from build123d import *

# Parameters (mm, degrees)
F1_DEPTH = 3


with BuildPart() as f1:
    # F0 (on Top) → F1 (new body)
    with BuildSketch(Plane.XY):
        with BuildLine():
            Line((-21, 3.2), (-21, 0))
            ThreePointArc((-21, 0), (-20.124574, -6.000127), (-17.571283, -11.5))
            ThreePointArc((-17.571283, -11.5), (-13.499794, -16.085881), (-8.277077, -19.3))
            Line((-8.277077, -19.3), (8.277077, -19.3))
            ThreePointArc((8.277077, -19.3), (13.499794, -16.085881), (17.571283, -11.5))
            ThreePointArc((17.571283, -11.5), (20.124574, -6.000127), (21, 0))
            Line((21, 0), (19, 0))
            Line((19, 0), (19, 3.2))
            Line((19, 3.2), (11, 3.2))
            Line((11, 3.2), (11, 0))
            Line((11, 0), (3, 0))
            Line((3, 0), (3, 3.2))
            Line((3, 3.2), (-5, 3.2))
            Line((-5, 3.2), (-5, 0))
            Line((-5, 0), (-13, 0))
            Line((-13, 0), (-13, 3.2))
            Line((-13, 3.2), (-21, 3.2))
        make_face()
    extrude(amount=F1_DEPTH)


solid = f1.part
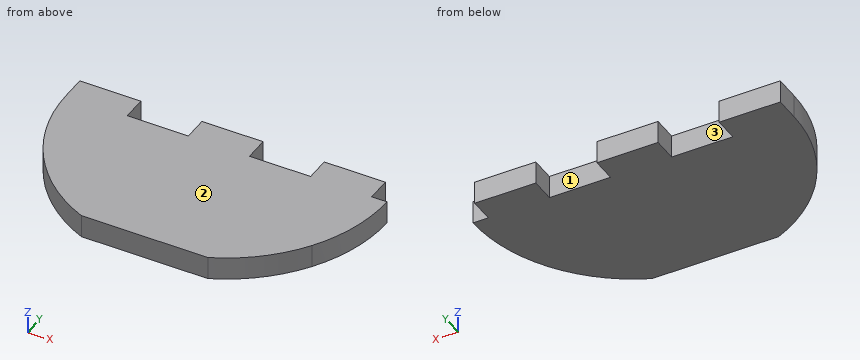
Verification items for the finished model (mm, model axes). Face numbers are marked on the shaded views. Coordinates: 2 decimals unless noted, no trailing zeros. Loops run counter-clockwise (first coordinate to the right, second up) from the corner with the lowest first, then second, coordinate; pieces in that order, holes last. Notation, with made-up numbers: (85.5, -1) -> (130.5, -1) arc R10 cw to (130.5, 12) -> close; hole circle Ø5 at (15.25, 83). An arc over 180 degrees is marked (long way). Answer as a JSON object with one key per item and string values. Group by question number.
Item 1: Sectioned sample at D-D on y = -16.5. Record the boundary of the cut face in (x, z), plus the area to 3 significant figures.
Item 2: Sectioned sample at A-A on y = 1.75. Record the boundary of the cut face in (x, z), plus the area to 3 significant figures.
Item 3: Mould release check, pull along X, two halves, no side actions. Record for the marked faces 1, 2 and 3: +X half, -X half, draft (parallel to the pull), parting line (faces both ways), or undercut.
Item 4: Depth check by flat-ended pin: pin 1 (1 mm diameter, centred on x = 20, z = 1, fed in from +Y). Enter the tip coordinate at first touch or a pass-through.
Item 5: Scan lines: probe 1 along Y at (x, z) = (7, 0.1); probe 2 along Y at (x, z) = (-17.5, 2.7); probe 3 along X at (y, z) = (-18, 2.05). Record each from-to range of solid material in increasing order.
Item 6: Sectioned sample at C-C on x = 4.5. Record the boundary of the cut face in (y, z), plus the area to 3 significant figures.
Item 7: Sectioned sample at B-B on z = 0.55. Record the boundary of the cut face in (x, y), plus the area to 3 significant figures.
Evaluation:
{
 "1": {"outline": "(-12.99, 0) -> (12.99, 0) -> (12.99, 3) -> (-12.99, 3) -> close", "area": "77.9 mm²"},
 "2": {"outline": "(-21, 0) -> (-13, 0) -> (-13, 3) -> (-21, 3) -> close; (-5, 0) -> (3, 0) -> (3, 3) -> (-5, 3) -> close; (11, 0) -> (19, 0) -> (19, 3) -> (11, 3) -> close", "area": "72.0 mm²"},
 "3": {"face 1": "undercut", "face 2": "draft", "face 3": "undercut"},
 "4": {"pin 1": "stops at y = 0"},
 "5": {"probe 1": "y = -19.3 to 0", "probe 2": "y = -11.61 to 3.2", "probe 3": "x = -10.82 to 10.82"},
 "6": {"outline": "(-19.3, 0) -> (0, 0) -> (0, 3) -> (-19.3, 3) -> close", "area": "57.9 mm²"},
 "7": {"outline": "(-21, 0) arc R21 ccw to (-17.57, -11.5) arc R21 ccw to (-8.28, -19.3) -> (8.28, -19.3) arc R21 ccw to (17.57, -11.5) arc R21 ccw to (21, 0) -> (19, 0) -> (19, 3.2) -> (11, 3.2) -> (11, 0) -> (3, 0) -> (3, 3.2) -> (-5, 3.2) -> (-5, 0) -> (-13, 0) -> (-13, 3.2) -> (-21, 3.2) -> close", "area": "751 mm²"}
}
